```python
from build123d import *

# Parameters (mm, degrees)
FILLET1_R = 0.33734375


with BuildPart() as part:
    # Sketch2 → Revolve1 (revolve)
    with BuildSketch(Plane.XY, mode=Mode.PRIVATE) as revolve1_sk:
        with BuildLine():
            Line((-5.953125, 0), (-5.953125, 13.15640625))
            ThreePointArc((-5.953125, 13.15640625), (-5.854319303, 13.394944303), (-5.61578125, 13.49375))
            Line((-5.61578125, 13.49375), (-3.175, 13.49375))
            Line((-3.175, 13.49375), (-3.175, 4.7625))
            Line((-3.175, 4.7625), (-1.7859375, 4.7625))
            Line((-1.7859375, 4.7625), (-1.7859375, 0))
            Line((-1.7859375, 0), (-5.953125, 0))
        make_face()
    revolve(revolve1_sk.sketch.rotate(Axis((0, 0, 0), (0, 1, 0)), 270), axis=Axis((0, 0, 0), (0, 1, 0)))

    # Fillet1
    fillet1_edges = [part.edges().sort_by_distance(p)[0] for p in [
        (0, 13.49375, 3.175),
    ]]
    fillet(fillet1_edges, radius=FILLET1_R)


solid = part.part
```
CAD build for the part. Positions are in the model's coordinates, mm. A direction names the side the tool comes from. Coordinates: 2 decimals unless noted, no trailing zeros. Order: outer loops, then holes, each group sorted by start corner. A loop starts at its lowest first (then second) coordinate and runs counter-clockwise, first axis right, second up.
(1) Which spindle directions (+Z, -Z, +X, -X, +Y, -Y) get a long thin tool onto all of the face, cutting with end or side? Do faces 5 (the face through (1.4, 4.762, -1.4)), 6 (the face through (4, 13.494, 0)). Say none if no direction does.
Solution:
face 5: +Y
face 6: +Z, -Z, +X, -X, +Y
(2) Drill centre lines: L1, parallel to X at y = 1.3, z = 0; L2, parallel to X at y = 9, z = 0 (3 decimals); L3, parallel to Y at x = -1.25, z = 1.5. Where is each one in solid material? Low to high.
Solution:
L1: x = -5.95 to -1.79, 1.79 to 5.95
L2: x = -5.953 to -3.175, 3.175 to 5.953
L3: y = 0 to 4.76
(3) Saw through at C-C, the plane y = 7. Write the cut outline in (x, z) (3 decimals).
Solution:
outline: circle Ø11.906 at (0, 0); hole circle Ø6.35 at (0, 0)
(4) Saw through at A-A, the plane x = 0. Write the cut outline in (y, z) (1 decimal), and give its area (3 significant figures).
Solution:
outline: (0, -6) - (13.2, -6) arc R0.3 ccw to (13.5, -5.6) - (13.5, -3.5) arc R0.3 ccw to (13.2, -3.2) - (4.8, -3.2) - (4.8, -1.8) - (0, -1.8) - close; (0, 1.8) - (4.8, 1.8) - (4.8, 3.2) - (13.2, 3.2) arc R0.3 ccw to (13.5, 3.5) - (13.5, 5.6) arc R0.3 ccw to (13.2, 6) - (0, 6) - close
area: 88.1 mm2
(5) Mould opens along Z. For faces 1 (the face through (1.93, 8.9, 2.52)), 2 (the face through (-1.4, 0, -1.4)), 3 (the face through (-0.079, 2.348, 1.784)), 4 (the face through (5.81, 6.67, 1.29)) say: released by +Z, released by -Z, zero draft, split by the parting line, or undercut.
Solution:
face 1: undercut
face 2: zero draft
face 3: undercut
face 4: split by the parting line
(6) Saw through at D-D, the plane y = 4. Write the cut outline in (x, z), and give its area (3 significant figures).
Solution:
outline: circle Ø11.91 at (0, 0); hole circle Ø3.57 at (0, 0)
area: 101 mm2
(7) Saw through at B-B, the plane z = 0. Write the cut outline in (x, y) (1 decimal).
Solution:
outline: (-6, 0) - (-1.8, 0) - (-1.8, 4.8) - (-3.2, 4.8) - (-3.2, 13.2) arc R0.3 ccw to (-3.5, 13.5) - (-5.6, 13.5) arc R0.3 ccw to (-6, 13.2) - close; (1.8, 0) - (6, 0) - (6, 13.2) arc R0.3 ccw to (5.6, 13.5) - (3.5, 13.5) arc R0.3 ccw to (3.2, 13.2) - (3.2, 4.8) - (1.8, 4.8) - close
(8) Pin check, flat tips, straight feed: pin 1 Ø3 at (x, z) = (0, 0) entering from -Y; pin 2 Ø5 at (y, z) = (5, 3) entering from -X; pin 3 Ø4 at (x, z) = (-1, -1) entering from -Y; pin 4 Ø1 at (x, y) = (-2, 11) entering from +Z. Stop position of each tip, or through.
Solution:
pin 1: passes through
pin 2: stops at x = -5.93
pin 3: stops at y = 0
pin 4: stops at z = 5.76
